Verification items for the finished model (mm, model axes). A direction names the side the tool comes from. Round coordinates to 2 decimals unless told otherwise and drop trailing zeros. Order: outer loops, then holes, each group sorted by start corner. A loop starts at its lowest first (then second) coordinate and runs counter-clockwise, first axis right, second up. Notation, with made-up numbers: (0, 51.5) -> (23, 51.5) arc R28 ccw to (23, 90.5) -> close; hole circle Ø11 at (53.5, -26). An arc over 180 degrees is marked (long way). Put each result on its own line as item: value.
Autodesk Inventor part; units mm, degrees
ref_plane "YZ Plane" through (0, 0, 0) normal (1, 0, 0) x (0, 1, 0)
ref_plane "XZ Plane" through (0, 0, 0) normal (0, 1, 0) x (-1, 0, 0)
ref_plane "XY Plane" through (0, 0, 0) normal (0, 0, 1) x (1, 0, 0)
sketch "Skizze1" plane through (0, 0, 0) normal (0, 0, 1) x (1, 0, 0)
  line L0 (0, 0) -> (20.5, 0) construction
  circle A0 centre (0, 0) radius 4
  arc A1 (8.6207, 9.0517) -> (12.5, 7.5) centre (12.5, 13.125) ccw
  arc A2 (12.5, -7.5) -> (8.6207, -9.0517) centre (12.5, -13.125) ccw
  line L1 (12.5, 7.5) -> (20.5, 7.5)
  line L2 (20.5, 7.5) -> (20.5, -7.5)
  line L3 (20.5, -7.5) -> (12.5, -7.5)
  line L4 (12.5, -7.5) -> (12.5, 7.5) construction
  circle A3 centre (0, 0) radius 10.5 construction
  line L5 (0, 0) -> (-10.5, 0) construction
  line L6 (16.5, 5.25) -> (16.5, -5.25) construction
  line L7 (16.5, 7.5) -> (16.5, -7.5) construction
  circle A4 centre (0, 0) radius 12.5
  point P0 (12.5, 0)
  point P1 (10.5, 0)
  point P2 (16.5, 0)
  dimension "d105" = 8
  dimension "d106" = 15
  dimension "LowerArm_ShaftFixation_Width" = 8
  dimension "d127" = 21
  dimension "d130" = 360
  dimension "d132" = 10.5
  dimension "d150" = 25
extrude "Grundprofil" add sketch "Skizze1" along normal blind 2
hole "Hole10" at (10.5, 0, 0) at (-10.5, 0, 0) direction (0, 0, 1) diameter 2.2 depth 12 tip angle 118 countersink diameter 4.4 countersink angle 90
hole "Hole11" at (16.5, 5.25, 0) at (16.5, -5.25, 0) direction (0, 0, 1) diameter 2.2 depth 3 tip angle 118 countersink diameter 4.4 countersink angle 90
properties part number "LowerArm_JointConnector_Prox_v2" material "Aluminum 6061"
Item 1: Sectioned sample at B-B, the plane y = 0. Record the boundary of the cut face in (x, z), then the cut area to 3 significant figures.
Geometry check:
outline: (-12.5, 0.2) -> (-11.6, 1.1) -> (-11.6, 2) -> (-12.5, 2) -> close; (-9.4, 1.1) -> (-8.3, 0) -> (-4, 0) -> (-4, 2) -> (-9.4, 2) -> close; (4, 0) -> (8.3, 0) -> (9.4, 1.1) -> (9.4, 2) -> (4, 2) -> close; (11.6, 1.1) -> (12.7, 0) -> (20.5, 0) -> (20.5, 2) -> (11.6, 2) -> close
area: 38.8 mm2
Item 2: Material ranges on line 1 along Y through (x, z) = (16.5, 1.4); line 2 along Y through (x, z) = (10.5, 1.5); line 3 along Y through (x, z) = (-10.5, 1.65), recorded low to high.
Geometry check:
line 1: -7.5 to -6.35, -4.15 to 4.15, 6.35 to 7.5
line 2: -7.87 to -1.1, 1.1 to 7.87
line 3: -6.78 to -1.1, 1.1 to 6.78
Item 3: Depth check by flat-ended pin: pin 1 Ø3.5 at (x, y) = (16.5, 5.25) entering from -Z; pin 2 Ø2.5 at (x, y) = (-10.5, 0) entering from -Z; pin 3 Ø1 at (x, z) = (14, 1) entering from +Y. Enter the tip coordinate at first touch or a pass-through.
Geometry check:
pin 1: z = 0.45
pin 2: z = 0.95
pin 3: y = 7.5
Item 4: Tool access check on faces 1 (the face through (10.44, 7.89, 0.99)), 2 (the face through (17, -7.5, 1)). Record the directions out of +Z, -Z, +X, -X, +Y, -Y that give a thin tool (end or side, any length) a straight path to the whole face; none if there is none.
Geometry check:
face 1: +Z, -Z, +X, +Y
face 2: +Z, -Z, +X, -Y
Item 5: Sectioned sample at A-A, the plane x = 16.5. Record the boundary of the cut face in (y, z).
Geometry check:
outline: (-7.5, 0) -> (-7.45, 0) -> (-6.35, 1.1) -> (-6.35, 2) -> (-7.5, 2) -> close; (-4.15, 1.1) -> (-3.05, 0) -> (3.05, 0) -> (4.15, 1.1) -> (4.15, 2) -> (-4.15, 2) -> close; (6.35, 1.1) -> (7.45, 0) -> (7.5, 0) -> (7.5, 2) -> (6.35, 2) -> close
Item 6: Sectioned sample at D-D, the plane x = 0. Record the boundary of the cut face in (y, z).
Geometry check:
outline: (-12.5, 0) -> (-4, 0) -> (-4, 2) -> (-12.5, 2) -> close; (4, 0) -> (12.5, 0) -> (12.5, 2) -> (4, 2) -> close
Item 7: Sectioned sample at C-C, the plane z = 1.5. Record the boundary of the cut face in (x, y), then the cut area to 3 significant figures.
Geometry check:
outline: (8.62, -9.05) arc R5.63 cw to (12.5, -7.5) -> (20.5, -7.5) -> (20.5, 7.5) -> (12.5, 7.5) arc R5.62 cw to (8.62, 9.05) arc R12.5 ccw (long way) to start; hole circle Ø2.2 at (-10.5, 0); hole circle Ø8 at (0, 0); hole circle Ø2.2 at (10.5, 0); hole circle Ø2.2 at (16.5, -5.25); hole circle Ø2.2 at (16.5, 5.25)
area: 559 mm2
Item 8: Release check for a two-part mould opening along Y. For faces 3 (the face through (17.574, 5.012, 1.556)), 4 (the face through (4, 3, 0)), 5 (the face through (16, 7.5, 1)) record: pulls with the +Y half, pulls with the -Y half, needs draft (parallel to the pull), parting line crosses it, or undercut.
Geometry check:
face 3: undercut
face 4: needs draft
face 5: pulls with the +Y half
